Model file for the job. Use its own axes, mm. Coordinates: 2 decimals unless noted, no trailing zeros. Order: outer loops, then holes, each group sorted by start corner. A loop starts at its lowest first (then second) coordinate and runs counter-clockwise, first axis right, second up. Notation, with made-up numbers: M 47.5,83.5 L 59.5,83.5 A14 ccw 59.5,101.5 Z; hole C 53.5,65 d3. An arc over 180 degrees is marked long. Return JSON: item names as keys, results as strings.
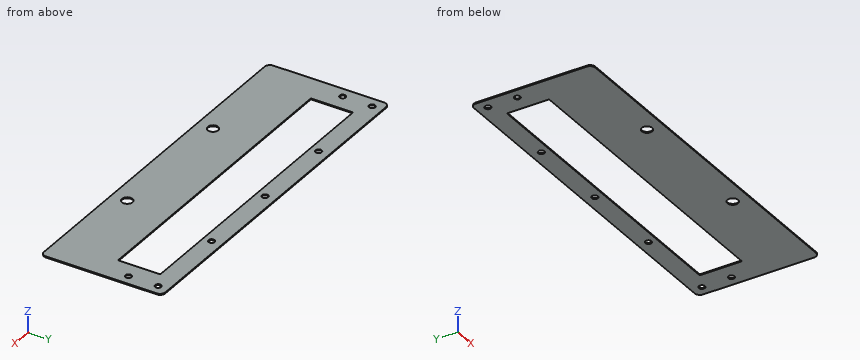
```python
from build123d import *

# Parameters (mm, degrees)
SKETCH1_W            = 342
SKETCH1_H            = 115
SKETCH1_W_2          = 290
SKETCH1_H_2          = 40
BOSS_EXTRUDE1_DEPTH  = 1
FILLET1_R            = 5
FILLET2_R            = 1
M5_CLEARANCE_HOLE1_D = 5.8
M8_CLEARANCE_HOLE1_D = 10


with BuildPart() as part:
    # Sketch1 → Boss-Extrude1 (new body)
    with BuildSketch(Plane.XY):
        Rectangle(SKETCH1_W, SKETCH1_H)
        with Locations((0, 19.5)):
            Rectangle(SKETCH1_W_2, SKETCH1_H_2, mode=Mode.SUBTRACT)
    extrude(amount=BOSS_EXTRUDE1_DEPTH)

    # Fillet1
    fillet1_edges = [part.edges().sort_by_distance(p)[0] for p in [
        (-171, 57.5, 0.5),
        (171, 57.5, 0.5),
        (171, -57.5, 0.5),
        (-171, -57.5, 0.5),
    ]]
    fillet(fillet1_edges, radius=FILLET1_R)

    # Fillet2
    fillet2_edges = [part.edges().sort_by_distance(p)[0] for p in [
        (-145, -0.5, 0.5),
        (145, -0.5, 0.5),
        (145, 39.5, 0.5),
        (-145, 39.5, 0.5),
    ]]
    fillet(fillet2_edges, radius=FILLET2_R)

    # M5 Clearance Hole1 (through all)
    with Locations(Plane.XY.offset(1)):
        with Locations((-161, 47.5), (-161, 19.5), (-80.5, 47.5), (0, 47.5), (80.5, 47.5), (161, 47.5), (161, 19.5)):
            Hole(M5_CLEARANCE_HOLE1_D / 2)

    # M8 Clearance Hole1 (through all)
    with Locations(Plane.XY.offset(1)):
        with Locations((-64.5, -42.5), (64.5, -42.5)):
            Hole(M8_CLEARANCE_HOLE1_D / 2)


solid = part.part
```
Item 1: Saw through at D-D (z = 0.7). Count the separate pieces of the cut face and the enclosed holes in it, and give its area (3 significant figures).
Check result:
{"separate pieces": "1", "enclosed holes": "10", "area": "27,400 mm2"}
Item 2: Saw through at B-B (y = 47.5). Write the cut outline in (x, z), and give its area (3 significant figures).
Check result:
{"outline": "M -171,0 L -163.9,0 L -163.9,1 L -171,1 Z; M -158.1,0 L -83.4,0 L -83.4,1 L -158.1,1 Z; M -77.6,0 L -2.9,0 L -2.9,1 L -77.6,1 Z; M 2.9,0 L 77.6,0 L 77.6,1 L 2.9,1 Z; M 83.4,0 L 158.1,0 L 158.1,1 L 83.4,1 Z; M 163.9,0 L 171,0 L 171,1 L 163.9,1 Z", "area": "313 mm2"}
Item 3: Saw through at C-C (x = -64.5). Write the cut outline in (y, z), and give its area (3 significant figures).
Check result:
{"outline": "M -57.5,0 L -47.5,0 L -47.5,1 L -57.5,1 Z; M -37.5,0 L -0.5,0 L -0.5,1 L -37.5,1 Z; M 39.5,0 L 57.5,0 L 57.5,1 L 39.5,1 Z", "area": "65.0 mm2"}
Item 4: Wall check: line 1 (Y direction, x = 161, z = 0.75); line 2 (Y direction, x = -64.5, z = 0.45); line 3 (Y direction, x = 97.5, z = 0.8). Give the ranges that are in metal, low to high.
Check result:
{"line 1": "y = -57.5 to 16.6, 22.4 to 44.6, 50.4 to 57.5", "line 2": "y = -57.5 to -47.5, -37.5 to -0.5, 39.5 to 57.5", "line 3": "y = -57.5 to -0.5, 39.5 to 57.5"}
Item 5: Saw through at A-A (x = -107). Write the cut outline in (y, z).
Check result:
{"outline": "M -57.5,0 L -0.5,0 L -0.5,1 L -57.5,1 Z; M 39.5,0 L 57.5,0 L 57.5,1 L 39.5,1 Z"}
